from build123d import *

# Parameters (mm, degrees)
SKETCH1_W           = 177.8
SKETCH1_H           = 69.85
BOSS_EXTRUDE1_DEPTH = 3.175
SKETCH2_R           = 3.175
CUT_EXTRUDE1_DEPTH  = 96.56697259
FILLET1_R           = 3.175
FILLET2_R           = 1.000000032
SKETCH3_R           = 1.74625
SKETCH3_R_2         = 8.255
CUT_EXTRUDE2_DEPTH  = 96.56697259


with BuildPart() as part:
    # Sketch1 → Boss-Extrude1 (new body)
    with BuildSketch(Plane(origin=(0, 0, 0), x_dir=(1, 0, 0), z_dir=(0, 1, 0))):
        Rectangle(SKETCH1_W, SKETCH1_H)
    extrude(amount=BOSS_EXTRUDE1_DEPTH)

    # Sketch2 → Cut-Extrude1 (cut, through all)
    with BuildSketch(Plane(origin=(0, 3.175, 0), x_dir=(1, 0, 0), z_dir=(0, 1, 0))):
        with Locations(Location((-82.55, 28.575, 0), (0, 0, 270))):
            Circle(SKETCH2_R)
        with Locations(Location((-82.55, -28.575, 0), (0, 0, 270))):
            Circle(SKETCH2_R)
        with Locations(Location((82.55, 28.575, 0), (0, 0, 270))):
            Circle(SKETCH2_R)
        with Locations(Location((82.55, -28.575, 0), (0, 0, 270))):
            Circle(SKETCH2_R)
    extrude(amount=-CUT_EXTRUDE1_DEPTH, mode=Mode.SUBTRACT)

    # Fillet1
    fillet1_edges = [part.edges().sort_by_distance(p)[0] for p in [
        (88.9, 1.5875, 34.925),
        (-88.9, 1.5875, 34.925),
        (-88.9, 1.5875, -34.925),
        (88.9, 1.5875, -34.925),
    ]]
    fillet(fillet1_edges, radius=FILLET1_R)

    # Fillet2
    fillet2_edges = [part.edges().sort_by_distance(p)[0] for p in [
        (0, 0, -34.925),
        (0, 3.175, -34.925),
        (88.9, 0, 0),
        (0, 0, 34.925),
        (-88.9, 0, 0),
        (-87.97006403, 0, 33.99506403),
        (-87.97006403, 0, -33.99506403),
        (87.97006403, 0, 33.99506403),
        (87.97006403, 0, -33.99506403),
        (88.9, 3.175, 0),
        (-88.9, 3.175, 0),
        (0, 3.175, 34.925),
        (-87.97006403, 3.175, 33.99506403),
        (-87.97006403, 3.175, -33.99506403),
        (87.97006403, 3.175, 33.99506403),
        (87.97006403, 3.175, -33.99506403),
    ]]
    fillet(fillet2_edges, radius=FILLET2_R)

    # Sketch3 → Cut-Extrude2 (cut, through all)
    with BuildSketch(Plane(origin=(0, 3.175, 0), x_dir=(1, 0, 0), z_dir=(0, 1, 0))):
        with Locations(Location((17.4625, 15.875, 0), (0, 0, 270))):
            Circle(SKETCH3_R)
        with Locations(Location((17.4625, -15.875, 0), (0, 0, 270))):
            Circle(SKETCH3_R)
        with Locations(Location((-17.4625, -15.875, 0), (0, 0, 270))):
            Circle(SKETCH3_R)
        with Locations(Location((-17.4625, 15.875, 0), (0, 0, 270))):
            Circle(SKETCH3_R)
        with Locations(Location((-63.5, 21.59, 0), (0, 0, 270))):
            Circle(SKETCH3_R_2)
        with Locations(Location((-38.1, 21.59, 0), (0, 0, 270))):
            Circle(SKETCH3_R_2)
        with Locations(Location((-38.1, 0, 0), (0, 0, 270))):
            Circle(SKETCH3_R_2)
        with Locations(Location((-63.5, 0, 0), (0, 0, 270))):
            Circle(SKETCH3_R_2)
        with Locations(Location((-38.1, -21.59, 0), (0, 0, 270))):
            Circle(SKETCH3_R_2)
        with Locations(Location((-63.5, -21.59, 0), (0, 0, 270))):
            Circle(SKETCH3_R_2)
        with Locations(Location((38.1, -21.59, 0), (0, 0, 270))):
            Circle(SKETCH3_R_2)
        with Locations(Location((63.5, -21.59, 0), (0, 0, 270))):
            Circle(SKETCH3_R_2)
        with Locations(Location((38.1, 0, 0), (0, 0, 270))):
            Circle(SKETCH3_R_2)
        with Locations(Location((63.5, 0, 0), (0, 0, 270))):
            Circle(SKETCH3_R_2)
        with Locations(Location((38.1, 21.59, 0), (0, 0, 270))):
            Circle(SKETCH3_R_2)
        with Locations(Location((63.5, 21.59, 0), (0, 0, 270))):
            Circle(SKETCH3_R_2)
    extrude(amount=-CUT_EXTRUDE2_DEPTH, mode=Mode.SUBTRACT)


solid = part.part
Work out the finished part from the listing and answer in its coordinate system (mm). Give positions to 0.01 mm unless a question says otherwise; leave off trailing zeros. Order: outer loops, then holes, each group sorted by start corner. A loop starts at its lowest first (then second) coordinate and runs counter-clockwise, first axis right, second up. Notation, with made-up numbers: (66, 44) -> (98, 44) arc R27 cw to (98, 82) -> close; hole circle Ø4 at (60, 66.5). An arc over 180 degrees is marked (long way). Answer as a JSON object with one key per item and string values. Group by question number.
1. Section D-D on z = -5 is taken. Determine the outline of the cut face in (x, y) (3 decimals).
2. Section C-C on x = -38.1 is taken. Determine the outline of the cut face in (y, z) (3 decimals), plus the area to 3 significant figures.
3. Section B-B on z = -21.59 is taken. Determine the outline of the cut face in (x, y) (3 decimals).
4. The mould has two halves that part along Z. Classify faces 1 (the cylindrical face through (30.04, 1.61, -1.79)), 2 (the cylindrical face through (-87.995, 1.596, 33.97)), 3 (the flat face through (-1, 0, 0)): released by +Z, released by -Z, zero draft, split by the parting line, or undercut.
5. Consider line 1 along X through (y, z) = (1.05, 21.59) (3 decimals); line 2 along X through (y, z) = (2.65, -7.5); line 3 along Z through (x, y) = (-64.5, 0.75). Determine where each line is inside the solid, lowest interval first. Write a range as [from, to].
6. Section A-A on x = 82.55 is taken. Determine the outline of the cut face in (y, z) (3 decimals), plus the area to 3 significant figures.
Result sheet:
{
 "1": {"outline": "(-88.9, 1) arc R1 ccw to (-87.9, 0) -> (-70.068, 0) -> (-70.068, 3.175) -> (-87.9, 3.175) arc R1 ccw to (-88.9, 2.175) -> close; (-56.932, 0) -> (-44.668, 0) -> (-44.668, 3.175) -> (-56.932, 3.175) -> close; (-31.532, 0) -> (31.532, 0) -> (31.532, 3.175) -> (-31.532, 3.175) -> close; (44.668, 0) -> (56.932, 0) -> (56.932, 3.175) -> (44.668, 3.175) -> close; (70.068, 0) -> (87.9, 0) arc R1 ccw to (88.9, 1) -> (88.9, 2.175) arc R1 ccw to (87.9, 3.175) -> (70.068, 3.175) -> close"},
 "2": {"outline": "(0, -33.925) arc R1 ccw to (1, -34.925) -> (2.175, -34.925) arc R1 ccw to (3.175, -33.925) -> (3.175, -29.845) -> (0, -29.845) -> close; (0, -13.335) -> (3.175, -13.335) -> (3.175, -8.255) -> (0, -8.255) -> close; (0, 8.255) -> (3.175, 8.255) -> (3.175, 13.335) -> (0, 13.335) -> close; (0, 29.845) -> (3.175, 29.845) -> (3.175, 33.925) arc R1 ccw to (2.175, 34.925) -> (1, 34.925) arc R1 ccw to (0, 33.925) -> close", "area": "63.7 mm^2"},
 "3": {"outline": "(-88.9, 1) arc R1 ccw to (-87.9, 0) -> (-71.755, 0) -> (-71.755, 3.175) -> (-87.9, 3.175) arc R1 ccw to (-88.9, 2.175) -> close; (-55.245, 0) -> (-46.355, 0) -> (-46.355, 3.175) -> (-55.245, 3.175) -> close; (-29.845, 0) -> (29.845, 0) -> (29.845, 3.175) -> (-29.845, 3.175) -> close; (46.355, 0) -> (55.245, 0) -> (55.245, 3.175) -> (46.355, 3.175) -> close; (71.755, 0) -> (87.9, 0) arc R1 ccw to (88.9, 1) -> (88.9, 2.175) arc R1 ccw to (87.9, 3.175) -> (71.755, 3.175) -> close"},
 "4": {"face 1": "undercut", "face 2": "released by +Z", "face 3": "zero draft"},
 "5": {"line 1": "x = [-88.9, -71.755], [-55.245, -46.355], [-29.845, 29.845], [46.355, 55.245], [71.755, 88.9]", "line 2": "x = [-88.78, -66.95], [-60.05, -41.55], [-34.65, 34.65], [41.55, 60.05], [66.95, 88.78]", "line 3": "z = [-34.89, -29.78], [-13.4, -8.19], [8.19, 13.4], [29.78, 34.89]"},
 "6": {"outline": "(0, -33.925) arc R1 ccw to (1, -34.925) -> (2.175, -34.925) arc R1 ccw to (3.175, -33.925) -> (3.175, -31.75) -> (0, -31.75) -> close; (0, -25.4) -> (3.175, -25.4) -> (3.175, 25.4) -> (0, 25.4) -> close; (0, 31.75) -> (3.175, 31.75) -> (3.175, 33.925) arc R1 ccw to (2.175, 34.925) -> (1, 34.925) arc R1 ccw to (0, 33.925) -> close", "area": "181 mm^2"}
}
